Autodesk Inventor part; units mm, degrees
ref_plane "YZ Plane" through (0, 0, 0) normal (1, 0, 0) x (0, 1, 0)
ref_plane "XZ Plane" through (0, 0, 0) normal (0, 1, 0) x (-1, 0, 0)
ref_plane "XY Plane" through (0, 0, 0) normal (0, 0, 1) x (1, 0, 0)
sketch "Skizze1" plane through (0, 0, 0) normal (0, 0, 1) x (1, 0, 0)
  line L0 (-12, 15) -> (51, 15)
  line L1 (52, 14) -> (52, -14)
  line L2 (51, -15) -> (-12, -15)
  line L3 (-13, -14) -> (-13, 14)
  arc A0 (-12, 15) -> (-13, 14) centre (-12, 14) ccw
  arc A1 (-13, -14) -> (-12, -15) centre (-12, -14) ccw
  arc A2 (51, -15) -> (52, -14) centre (51, -14) ccw
  arc A3 (52, 14) -> (51, 15) centre (51, 14) ccw
  point P0 (0, 0)
  point P1 (-13, 15)
  point P2 (52, 15)
  point P3 (-13, -15)
  dimension "d0" = 65
  dimension "d1" = 30
  dimension "d2" = 15
  dimension "d3" = 13
  dimension "d4" = 1
extrude "Extrusion1" add sketch "Skizze1" along normal blind 31
sketch "Skizze2" plane through (0, 0, 31) normal (0, 0, 1) x (1, 0, 0)
  line L0 (-20.5, 15) -> (59.5, 15)
  line L1 (59.5, -15) -> (-20.5, -15)
  arc A0 (-20.5, 15) -> (-21.5, 14) centre (-20.5, 14) ccw
  arc A1 (-21.5, -14) -> (-20.5, -15) centre (-20.5, -14) ccw
  arc A2 (59.5, -15) -> (60.5, -14) centre (59.5, -14) ccw
  arc A3 (60.5, 14) -> (59.5, 15) centre (59.5, 14) ccw
  arc A4 (-20.3995, 7.2) -> (-20.3995, 9.7) centre (-17.95, 8.45) ccw
  arc A5 (-20.3995, -9.7) -> (-20.3995, -7.2) centre (-17.95, -8.45) ccw
  line L2 (-20.3995, -7.2) -> (-21.5, -7.2)
  line L3 (-21.5, -9.7) -> (-20.3995, -9.7)
  line L4 (-21.5, -14) -> (-21.5, -9.7)
  line L5 (-20.3995, 9.7) -> (-21.5, 9.7)
  line L6 (-21.5, 7.2) -> (-20.3995, 7.2)
  line L7 (-21.5, -7.2) -> (-21.5, 7.2)
  line L8 (-21.5, 9.7) -> (-21.5, 14)
  line L9 (19.5, 16.9478) -> (19.5, -22.1923) construction
  arc A6 (59.3995, 9.7) -> (59.3995, 7.2) centre (56.95, 8.45) ccw
  arc A7 (59.3995, -7.2) -> (59.3995, -9.7) centre (56.95, -8.45) ccw
  line L10 (59.3995, -7.2) -> (60.5, -7.2)
  line L11 (60.5, -9.7) -> (59.3995, -9.7)
  line L12 (60.5, -14) -> (60.5, -9.7)
  line L13 (59.3995, 9.7) -> (60.5, 9.7)
  line L14 (60.5, 7.2) -> (59.3995, 7.2)
  line L15 (60.5, -7.2) -> (60.5, 7.2)
  line L16 (60.5, 9.7) -> (60.5, 14)
  point P0 (0, 0)
  point P1 (60.5, -15)
  point P2 (60.5, 15)
  dimension "d7" = 30
  dimension "d10" = 1
  dimension "d11" = 15
  dimension "d12" = 5.5
  dimension "d13" = 5.5
  dimension "d14" = 6.55
  dimension "d15" = 6.55
  dimension "d19" = 1.25
  dimension "d23" = 1.25
  dimension "d25" = 41
  dimension "d26" = 21.5
extrude "Extrusion2" add sketch "Skizze2" along normal blind 4
sketch "Skizze3" plane through (0, 0, 35) normal (0, 0, 1) x (1, 0, 0)
  line L0 (-12, 15) -> (51, 15)
  line L1 (52, 14) -> (52, -14)
  line L2 (51, -15) -> (-12, -15)
  line L3 (-13, -14) -> (-13, 14)
  arc A0 (-12, 15) -> (-13, 14) centre (-12, 14) ccw
  arc A1 (-13, -14) -> (-12, -15) centre (-12, -14) ccw
  arc A2 (51, -15) -> (52, -14) centre (51, -14) ccw
  arc A3 (52, 14) -> (51, 15) centre (51, 14) ccw
  point P0 (0, 0)
  point P1 (0, 0)
  point P2 (-13, 15)
  point P3 (52, 15)
  point P4 (-13, -15)
  dimension "d29" = 65
  dimension "d30" = 30
  dimension "d31" = 15
  dimension "d32" = 13
  dimension "d33" = 1
extrude "Extrusion3" add sketch "Skizze3" along normal blind 14
chamfer "Fase1" distance 4 angle 45 1 edges at (-13, 0, 49)
sketch "Skizze4" plane through (0, 0, 49) normal (0, 0, 1) x (1, 0, 0)
  circle A0 centre (0, 0) radius 4
  dimension "d39" = 8
extrude "Extrusion4" add sketch "Skizze4" along normal blind 7
properties part number "Servo"
Could you check a few things on this model? Use its own coordinates, in mm. A direction names the side the tool comes from. Give positions to 0.01 mm unless a question says otherwise; leave off trailing zeros. Write each loop counter-clockwise with the first axis right and the second up, starting at its lowest first coordinate (ties: lowest second). Pieces come first, ordered by that corner, then holes. Notation, with made-up numbers: (68.5, -38) -> (113.5, -38) arc R36 ccw to (113.5, 1) -> close; hole circle Ø7 at (65, -39). An arc over 180 degrees is marked (long way). Write each question's results on one line, items separated by ' | '. Start each with the question number.
Q1. Which directions (+Z, -Z, +X, -X, +Y, -Y) give clear straight access to the entire face, cutting with the end or side of a thin tool? Please do faces 1 (the face through (-13, 0, 15)), 2 (the face through (-13, 0, 40)), 3 (the face through (0, 0, 56)), 4 (the face through (52, 0, 42)).
Q2. Suppose I cut it at A-A, the plane x = 56.95. List the corners of the cut face in (y, z) for me.
Q3. I'm going to push flat-ended pins straight in: pin 1 Ø7 at (y, z) = (5.5, 40.5) entering from +X; pin 2 Ø3 at (x, y) = (-19, 0) entering from -Z; pin 3 Ø10.5 at (x, y) = (-18, -4) entering from +Z; pin 4 Ø10.5 at (x, y) = (55, 3.5) entering from -Z. Where does each tip first touch, or does it pass through?
Q4. We'd pull the mould along X, two halves only. Please class faces 5 (the face through (54.2, 8.35, 32.97)), 6 (the face through (-17, 0, 31)), 7 (the face through (-21.5, 12, 33)): +X half, -X half, draft (parallel to the pull), parting line (faces both ways), or undercut.
Q5. Suppose I cut it at B-B, the plane y = -12.5. List the corners of the cut face in (x, z) for me.
Q6. Suppose I cut it at C-C, the plane z = 12. List the corners of the cut face in (x, y) for me, and give its area (3 significant figures).
Q7. Suppose I cut it at D-D, the plane x = -10.5. List the corners of the cut face in (y, z) for me.
Q8. I need wall thicknesses on probe 1 along Y at (x, z) = (-17.95, 34.05); probe 2 along Y at (x, z) = (-17, 34); probe 3 along X at (y, z) = (-10, 32). Which ranges of each line are inside material? Lowest first, please.
Outcome:
1) face 1: -Z, -X, +Y, -Y | face 2: +Z, -X, +Y, -Y | face 3: +Z, +X, -X, +Y, -Y | face 4: +Z, +X, +Y, -Y
2) outline: (-15, 31) -> (-11.2, 31) -> (-11.2, 35) -> (-15, 35) -> close; (-5.7, 31) -> (5.7, 31) -> (5.7, 35) -> (-5.7, 35) -> close; (11.2, 31) -> (15, 31) -> (15, 35) -> (11.2, 35) -> close
3) pin 1: x = 52 | pin 2: z = 31 | pin 3: z = 45.25 | pin 4: z = 0
4) face 5: undercut | face 6: draft | face 7: -X half
5) outline: (-21.5, 31) -> (-13, 31) -> (-13, 0) -> (52, 0) -> (52, 31) -> (60.5, 31) -> (60.5, 35) -> (52, 35) -> (52, 49) -> (-9, 49) -> (-13, 45) -> (-13, 35) -> (-21.5, 35) -> close
6) outline: (-13, -14) arc R1 ccw to (-12, -15) -> (51, -15) arc R1 ccw to (52, -14) -> (52, 14) arc R1 ccw to (51, 15) -> (-12, 15) arc R1 ccw to (-13, 14) -> close | area: 1,950 mm2
7) outline: (-15, 0) -> (15, 0) -> (15, 47.5) -> (-15, 47.5) -> close
8) probe 1: -15 to -11.2, -5.7 to 5.7, 11.2 to 15 | probe 2: -15 to -11.03, -5.87 to 5.87, 11.03 to 15 | probe 3: -21.5 to -20.22, -15.68 to 54.68, 59.22 to 60.5
